Can you work these out from the model? Positions are in its coordinate system, mm. Face numbers are marked on the shaded views. A direction names the side the tool comes from. Give positions to 0.01 mm unless a question says otherwise; leave off trailing zeros. Loops run counter-clockwise (first coordinate to the right, second up) from the corner with the lowest first, then second, coordinate; pieces in that order, holes last. Notation, with made-up numbers: M -15,-2 L 1,-2 A21 cw 1,31 Z; hole C 19.5,85.5 d2. An arc over 180 degrees is marked long. Answer as a JSON object with one key per item and string values.
```python
from build123d import *

# Parameters (mm, degrees)
F0_W     = 76.2
F0_H     = 76.2
F3_DEPTH = 6.35
F6_E7_W  = 76.2
F6_E7_H  = 25.4
F7_DEPTH = 2.00000108
F6_E9_W  = 76.2
F6_E9_H  = 25.4
F8_DEPTH = 2.00000108
F5_E11_W = 76.2
F5_E11_H = 25.4
F5_E5_W  = 76.2
F5_E5_H  = 25.4
F9_DEPTH = 2.00000108


# Not quite as in the source:
# - the program builds the solid bodies; features that only make, move or delete a surface that nothing else refers to are left out


with BuildPart() as f3:
    # F0 (on Front) → F3 (new body)
    with BuildSketch(Plane.XZ):
        with Locations((-0.0921785831, 11.5903750752)):
            Rectangle(F0_W, F0_H)
    extrude(amount=F3_DEPTH)

    # F6_E7 (on explicit) → F7 (join)
    with BuildSketch(Plane(origin=(-38.1921785831, 0, 25.7983756152), x_dir=(1, 0, 0), z_dir=(0, 0, -1))):
        with Locations((38.1, 12.7)):
            Rectangle(F6_E7_W, F6_E7_H)
    extrude(amount=F7_DEPTH)

    # F6_E9 (on explicit) → F8 (join)
    with BuildSketch(Plane(origin=(-38.1921785831, 0, -0.6176243848), x_dir=(1, 0, 0), z_dir=(0, 0, -1))):
        with Locations((38.1, 12.7)):
            Rectangle(F6_E9_W, F6_E9_H)
    extrude(amount=F8_DEPTH)

    # F5_E11 (on explicit) + F5_E5 (on explicit) → F9 (join)
    with BuildSketch(Plane(origin=(-12.2921770431, 0, 49.6903750752), x_dir=(0, 0, -1), z_dir=(-1, 0, 0))):
        with Locations((38.1, 12.7)):
            Rectangle(F5_E11_W, F5_E11_H)
    with BuildSketch(Plane(origin=(14.1078209569, 0, 49.6903750752), x_dir=(0, 0, -1), z_dir=(-1, 0, 0))):
        with Locations((38.1, 12.7)):
            Rectangle(F5_E5_W, F5_E5_H)
    extrude(amount=F9_DEPTH)


solid = f3.part
```
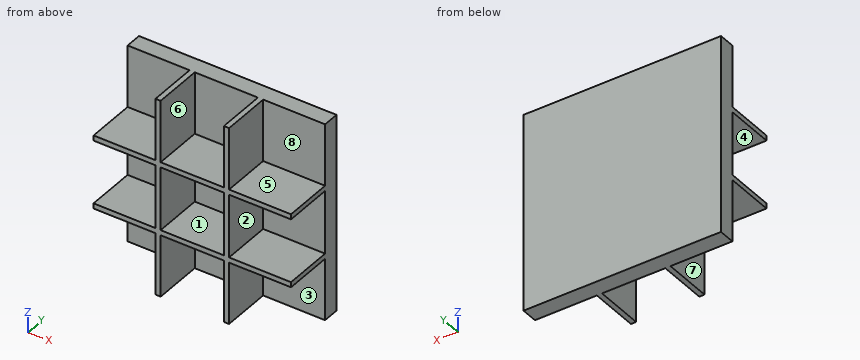
1) Will these pins go through, and if not, where does the flat tip stop? pin 1 Ø5.5 at (x, y) = (-22.5, -14.5) entering from -Z; pin 2 Ø5 at (y, z) = (-10.5, 8.5) entering from -X; pin 3 Ø12 at (x, z) = (26, -16.5) entering from -Y.
Answer list:
{"pin 1": "z = -2.62", "pin 2": "x = -14.29", "pin 3": "y = -6.35"}
2) For the marked faces 1, 2, 3, 4 and 5, which set-ups out of +Z, -Z, +X, -X, +Y, -Y let a thin tool reach every point of the face, with its end or its side?
Answer list:
{"face 1": "-Y", "face 2": "+X, -Y", "face 3": "-Z, +X, -Y", "face 4": "-X, -Y", "face 5": "+Z, +X, -Y"}
3) Please list where these lines run through material, in increasing order: line 1 along X through (y, z) = (-9.5, 1.5); line 2 along Z through (x, y) = (-28, -15); line 3 along Y through (x, z) = (-1.5, -21). Write a range as from..to.
Answer list:
{"line 1": "-14.29..-12.29, 12.11..14.11", "line 2": "-2.62..-0.62, 23.8..25.8", "line 3": "-6.35..0"}
4) Suppose I cut it at C-C, the plane x = -7. Write out the boundary of the cut face in (y, z).
Answer list:
{"outline": "M -25.4,-2.62 L -6.35,-2.62 L -6.35,-26.51 L 0,-26.51 L 0,49.69 L -6.35,49.69 L -6.35,25.8 L -25.4,25.8 L -25.4,23.8 L -6.35,23.8 L -6.35,-0.62 L -25.4,-0.62 Z"}
5) Suppose I cut it at B-B, the plane z = 45.5. Write out the boundary of the cut face in (x, y).
Answer list:
{"outline": "M -38.19,-6.35 L -14.29,-6.35 L -14.29,-25.4 L -12.29,-25.4 L -12.29,-6.35 L 12.11,-6.35 L 12.11,-25.4 L 14.11,-25.4 L 14.11,-6.35 L 38.01,-6.35 L 38.01,0 L -38.19,0 Z"}
6) If we mould it in two halves opening along X, with no side actions, what happens to the marked faces 6, 7 and 8? For each: +X half, -X half, draft (parallel to the pull), parting line (faces both ways), or undercut.
Answer list:
{"face 6": "undercut", "face 7": "-X half", "face 8": "draft"}
